from build123d import *

# Parameters (mm, degrees)
F0_W     = 30
F0_H     = 10
F1_DEPTH = 5
F3_DEPTH = 25
F4_DEPTH = 18
F5_R     = 5
F6_R     = 2


with BuildPart() as f1:
    # F0 (on Top) → F1 (new body)
    with BuildSketch(Plane.XY):
        with Locations((0.6170257553, -0.1298129745)):
            Rectangle(F0_W, F0_H)
    extrude(amount=F1_DEPTH)

    # F2 (on face) → F3 (join)
    with BuildSketch(Plane.XY.offset(5)):
        Polygon((15.6170257553, 4.8701870255), (-14.3829742447, 4.8701870255), (-14.3829742447, 2.8308965266), (-11.7144621909, 2.8308965266), (12.1078416705, 2.8308965266), (15.6170257553, 2.8308965266), align=None)
    extrude(amount=F3_DEPTH)

    # F2 (on face) → F4 (join)
    with BuildSketch(Plane.XY.offset(5)):
        Polygon((-11.7144621909, 2.8308965266), (-14.3829742447, 2.8308965266), (-14.3829742447, -5.1298129745), (-5.2125030197, -5.1298129745), (-5.2125030197, -2.4143811315), (-11.7144621909, -2.4143811315), align=None)
        Polygon((15.6170257553, -5.1298129745), (15.6170257553, 2.8308965266), (12.1078416705, 2.8308965266), (12.1078416705, -2.4143811315), (5.6058824994, -2.4143811315), (5.6058824994, -5.1298129745), align=None)
    extrude(amount=F4_DEPTH)

    # F5
    f5_edges = [f1.edges().sort_by_distance(p)[0] for p in [
        (-5.212503, -3.772097, 23),
        (5.605882, -3.772097, 23),
    ]]
    fillet(f5_edges, radius=F5_R)

    # F6
    f6_edges = [f1.edges().sort_by_distance(p)[0] for p in [
        (0.617026, 2.830897, 30),
        (15.617026, -0.129813, 0),
        (15.617026, -1.149458, 23),
        (-14.382974, -1.149458, 23),
        (-14.382974, -0.129813, 0),
    ]]
    fillet(f6_edges, radius=F6_R)


solid = f1.part
Could you check a few things on this model? Use its own coordinates, in mm. A direction names the side the tool comes from. Give positions to 0.01 mm unless a question says otherwise; leave off trailing zeros. Order: outer loops, then holes, each group sorted by start corner. A loop starts at its lowest first (then second) coordinate and runs counter-clockwise, first axis right, second up. Notation, with made-up numbers: (75, 15) -> (125, 15) arc R23 cw to (125, 26) -> close; hole circle Ø8 at (87, -28). An arc over 180 degrees is marked (long way). Answer in a Markdown table with one row per item. Add a question column.
Item 1: We'd pull the mould along Y, two halves only. Please class faces 4 (the cylindrical face through (15.016, -0.06, 0.57)), 5 (the flat face through (0, -5.13, 4)), 6 (the flat face through (-11.714, 0, 14)): pulls with the +Y half, pulls with the -Y half, needs draft (parallel to the pull), parting line crosses it, or undercut.
Item 2: Imagine slicing it at B-B (y = -4). List the corners of the cut face in (x, z) for me, and give its area (3 significant figures).
Item 3: I'm going to push flat-ended pins straight in: P1, Ø2, axis at x = -7, y = -3, coming from the +Z side; P2, Ø1.5, axis at y = -1, z = 23.5, coming from the +X side; P3, Ø1.5, axis at x = 12.5, y = -1, coming from the +Z side. Where does each tip first touch, or does it pass through?
Item 4: For faces 1 (the flat face through (5.606, -4, 11)), 2 (the cylindrical face through (-13.78, -1.21, 22.43)), 3 (the flat face through (-8, -2.414, 14)), which set-ups out of +Z, -Z, +X, -X, +Y, -Y let a thin tool reach every point of the face, with its end or its side?
Item 5: Imagine slicing it at C-C (z = 13.5). List the corners of the cut face in (x, y) for me, and give its area (3 significant figures).
Item 6: Please list where these lines run through material, in increasing order: probe 1 along X at (y, z) = (-4.25, 17); probe 2 along Y at (x, z) = (8.25, 21.25); probe 3 along X at (y, z) = (2, 10).
Result:
| question | item | result |
|---|---|---|
| 1 | face 4 | needs draft |
| 1 | face 5 | pulls with the -Y half |
| 1 | face 6 | undercut |
| 2 | outline | (-14.38, 2) arc R2 ccw to (-12.38, 0) -> (13.62, 0) arc R2 ccw to (15.62, 2) -> (15.62, 21) arc R2 ccw to (13.62, 23) -> (10.61, 23) arc R5 ccw to (5.61, 18) -> (5.61, 5) -> (-5.21, 5) -> (-5.21, 18) arc R5 ccw to (-10.21, 23) -> (-12.38, 23) arc R2 ccw to (-14.38, 21) -> close |
| 2 | area | 481 mm2 |
| 3 | P1 | z = 22.48 |
| 3 | P2 | x = 14.59 |
| 3 | P3 | z = 23 |
| 4 | face 1 | +Z, -Y |
| 4 | face 2 | +Z, -X, -Y |
| 4 | face 3 | +Z |
| 5 | outline | (-14.38, -5.13) -> (-5.21, -5.13) -> (-5.21, -2.41) -> (-11.71, -2.41) -> (-11.71, 2.83) -> (12.11, 2.83) -> (12.11, -2.41) -> (5.61, -2.41) -> (5.61, -5.13) -> (15.62, -5.13) -> (15.62, 4.87) -> (-14.38, 4.87) -> close |
| 5 | area | 146 mm2 |
| 6 | probe 1 | -14.38 to -5.21, 5.61 to 15.62 |
| 6 | probe 2 | -5.13 to -2.41, 2.83 to 4.87 |
| 6 | probe 3 | -14.38 to -11.71, 12.11 to 15.62 |
